Autodesk Inventor part; units mm, degrees
ref_plane "YZ Plane" through (0, 0, 0) normal (1, 0, 0) x (0, 1, 0)
ref_plane "XZ Plane" through (0, 0, 0) normal (0, 1, 0) x (-1, 0, 0)
ref_plane "XY Plane" through (0, 0, 0) normal (0, 0, 1) x (1, 0, 0)
sketch "Sketch1" plane through (0, 0, 0) normal (0, 1, 0) x (-1, 0, 0)
  line L0 (0, 0) -> (34.163, 0)
  line L1 (34.163, 0) -> (34.163, -22.098)
  line L2 (34.163, -22.098) -> (0, -22.098)
  line L3 (0, -22.098) -> (0, 0)
  dimension "d0" = 34.163
  dimension "d1" = 22.098
extrude "Extrusion1" add sketch "Sketch1" along normal blind 1.5748
hole "Hole2" at (-10.9855, 1.5748, -3.4925) direction (0, -1, 0) diameter 3.175 depth 25.4 tip angle 118
hole "Hole3" at (-10.9855, 1.5748, -18.6055) direction (0, -1, 0) diameter 3.175 depth 25.4 tip angle 118
properties part number "temp_probe_board"
The listing builds one solid part. Answer for the finished solid, in the listing's coordinates (mm). Give positions to 0.01 mm unless a question says otherwise; leave off trailing zeros. Order: outer loops, then holes, each group sorted by start corner. A loop starts at its lowest first (then second) coordinate and runs counter-clockwise, first axis right, second up. Notation, with made-up numbers: (-8, -0.75) - (1, -0.75) arc R20 cw to (1, 24.25) - close; hole circle Ø4 at (-37, 55.5). An arc over 180 degrees is marked (long way). Answer in a Markdown table with one row per item. Add a question column.
Q1. For a pull along Z with two mould halves and no side action, classify faces 1 (the flat face through (-17, 1, 0)), 2 (the cylindrical face through (-10.02, 0.776, -4.752)), 3 (the flat face through (-17, 0, -11)) as released by +Z, released by -Z, zero draft, split by the parting line, or undercut.
Q2. Given P1, Ø3, axis at x = -10.99, z = -18.61, coming from the +Y side, flat-ended and moving along its own axis, determine where the tip first touches the part or whether it passes through.
Q3. The part is cut by section A-A (z = -4.5). Determine the outline of the cut face in (x, y).
Q4. The part is cut by section B-B (y = 1.25). Determine the outline of the cut face in (x, z) (1 decimal), then the cut area to 3 significant figures.
Q5. Find the intervals of material crossed by line 1 along X through (y, z) = (0.35, -20); line 2 along X through (y, z) = (0.8, -19.5), in increasing order. Write a range as [from, to].
Determined:
| question | item | result |
|---|---|---|
| 1 | face 1 | released by +Z |
| 1 | face 2 | undercut |
| 1 | face 3 | zero draft |
| 2 | P1 | passes through |
| 3 | outline | (-34.16, 0) - (-12.21, 0) - (-12.21, 1.57) - (-34.16, 1.57) - close; (-9.76, 0) - (0, 0) - (0, 1.57) - (-9.76, 1.57) - close |
| 4 | outline | (-34.2, -22.1) - (0, -22.1) - (0, 0) - (-34.2, 0) - close; hole circle Ø3.2 at (-11, -18.6); hole circle Ø3.2 at (-11, -3.5) |
| 4 | area | 739 mm² |
| 5 | line 1 | x = [-34.16, -11.74], [-10.23, 0] |
| 5 | line 2 | x = [-34.16, -12.3], [-9.67, 0] |
